Geometry check sheet. Reference: the model listing, model coordinates, mm. A direction names the side the tool comes from. Coordinates: 2 decimals unless noted, no trailing zeros. Loops run counter-clockwise (first coordinate to the right, second up) from the corner with the lowest first, then second, coordinate; pieces in that order, holes last.
Autodesk Inventor part; units mm, degrees
ref_plane "bolt_XY" through (0, 0, 0) normal (1, 0, 0) x (0, 0, -1)
ref_plane "bolt_YZ" through (0, 0, 0) normal (0, 0, -1) x (0, 1, 0)
ref_plane "bolt_ZX" through (0, 0, 0) normal (0, 1, 0) x (1, 0, 0)
sketch "Sketch_1" plane through (0, 0, 0) normal (0, 0, 1) x (1, 0, 0)
  line L0 (20, 0) -> (-4, 0)
  line L1 (-4, 0) -> (-4, 3.5)
  line L2 (-4, 3.5) -> (0, 3.5)
  line L3 (0, 3.5) -> (0, 2)
  line L4 (0, 2) -> (19.5705, 2)
  line L5 (19.5705, 2) -> (20, 1.5705)
  line L6 (20, 1.5705) -> (20, 0)
  line L7 (20, 0) -> (-4, 0)
revolve "Revolution1" add sketch "Sketch_1" angle 360 about axis through (20, 0, 0) along (1, 0, 0)
thread "Thread1"
sketch "Sketch_4" plane through (0, 0, 0) normal (0, 0, 1) x (1, 0, 0)
  line L0 (-1.5981, 0) -> (-4, 0)
  line L1 (-4, 0) -> (-4, 1.5)
  line L2 (-4, 1.5) -> (-2, 1.5)
  line L3 (-2, 1.5) -> (-1.5981, 0)
  line L4 (-1.5981, 0) -> (-4, 0)
revolve "Revolution2" cut sketch "Sketch_4" angle 360 about axis through (-1.5981, 0, 0) along (1, 0, 0)
sketch "Sketch_3" plane through (-4, 0, 0) normal (1, 0, 0) x (0, 0, -1)
  line L0 (-1.5, 0.866) -> (-1.5, -0.866)
  line L1 (-1.5, -0.866) -> (0, -1.7321)
  line L2 (0, -1.7321) -> (1.5, -0.866)
  line L3 (1.5, -0.866) -> (1.5, 0.866)
  line L4 (1.5, 0.866) -> (0, 1.7321)
  line L5 (0, 1.7321) -> (-1.5, 0.866)
extrude "Extrusion1" cut sketch "Sketch_3" along normal blind 2
ref_plane "bolt_XY" through (0, 0, 0) normal (1, 0, 0) x (0, 0, -1)
ref_plane "bolt_YZ" through (0, 0, 0) normal (0, 0, -1) x (0, 1, 0)
ref_plane "bolt_ZX" through (0, 0, 0) normal (0, 1, 0) x (1, 0, 0)
ref_plane "nut_XY" through (20, 0, 0) normal (1, 0, 0) x (0, 0, -1)
ref_plane "nut_YZ" through (20, 0, 0) normal (0, 0, -1) x (0, 1, 0)
ref_plane "nut_ZX" through (20, 0, 0) normal (0, 1, 0) x (1, 0, 0)
properties part number "CBM4-20" material "MISUMI"
1) Section check B-B on y = 2.75. Record the cut outline in (x, z).
Data:
outline: (-4, -2.17) - (0, -2.17) - (0, 2.17) - (-4, 2.17) - close
2) Access from +Z, -Z, +X, -X, +Y, -Y to the whole of each face (thin tool, end or side, straight path). Record for faces 4 (the flat face through (20, 0, 0)), 5 (the cylindrical face through (10, 0, -2)), 6 (the flat face through (-3.014, -1.293, 0.76)).
Data:
face 4: +Z, -Z, +X, +Y, -Y
face 5: +X
face 6: -X
3) Material ranges on probe 1 along Z at (x, y) = (4.5, -1); probe 2 along X at (y, z) = (-2, 1.75); probe 3 along Y at (x, z) = (-2.25, -0.5), recorded low to high.
Data:
probe 1: z = -1.73 to 1.73
probe 2: x = -4 to 0
probe 3: y = -3.46 to -1.44, 1.44 to 3.46
4) Mould release check, pull along Z, two halves, no side actions. Record for faces 1 (the conical face through (-1.623, -0.02, 0.092)), 2 (the cylindrical face through (-1.972, 3.233, -1.341)), 3 (the flat face through (0, 2, -2)): +Z half, -Z half, draft (parallel to the pull), parting line (faces both ways), or undercut.
Data:
face 1: undercut
face 2: parting line
face 3: draft
5) Section check A-A on x = 14.25. Record the cut outline in (y, z), and give its area (3 significant figures).
Data:
outline: circle Ø4 at (0, 0)
area: 12.6 mm2
6) Section check C-C on z = -2.25. Record the cut outline in (x, y).
Data:
outline: (-4, -2.68) - (0, -2.68) - (0, 2.68) - (-4, 2.68) - close
7) Depth check by flat-ended pin: pin 1 (1 mm diameter, centred on x = 2.5, z = 1.5, fed in from +Y); pin 2 (0.5 mm diameter, centred on y = -0.5, z = 0.5, fed in from -X); pin 3 (1 mm diameter, centred on x = 4, z = -2, fed in from -Y). Enter the tip coordinate at first touch or a pass-through.
Data:
pin 1: stops at y = 1.73
pin 2: stops at x = -1.85
pin 3: stops at y = -1.32
